Can you work these out from the model? Positions are in its coordinate system, mm. Face numbers are marked on the shaded views. Give positions to 0.01 mm unless a question says otherwise; leave off trailing zeros. Order: outer loops, then holes, each group sorted by start corner. A loop starts at its lowest first (then second) coordinate and runs counter-clockwise, first axis right, second up. Notation, with made-up numbers: M 56.5,13.5 L 110.5,13.5 A25 ccw 110.5,30.5 Z; hole C 19,19 d8. An arc over 180 degrees is marked long. Answer as a JSON object with one key per item and string values.
```python
from build123d import *

# Parameters (mm, degrees)
PAD_DEPTH    = 10
CHAMFER_SIZE = 1


with BuildPart() as part:
    # Sketch → Pad (new body)
    with BuildSketch(Plane.XY):
        with BuildLine():
            Line((-0.8, 8), (-0.8, 0))
            Line((-0.8, 0), (0.8, 0))
            Line((0.8, 8), (0.8, 0))
            ThreePointArc((3.222844, 7.624292), (2.025901, 7.905515), (0.8, 8))
            Line((3.222844, 7.624292), (68.028555, -12.969635))
            ThreePointArc((75, -22.5), (73.071107, -16.595999), (68.028555, -12.969635))
            Line((75, -22.5), (65, -22.5))
            ThreePointArc((65, -22.5), (0, -10), (-65, -22.5))
            Line((-75, -22.5), (-65, -22.5))
            ThreePointArc((-68.028555, -12.969635), (-73.071107, -16.595999), (-75, -22.5))
            Line((-3.222844, 7.624292), (-68.028555, -12.969635))
            ThreePointArc((-0.8, 8), (-2.025901, 7.905515), (-3.222844, 7.624292))
        make_face()
    extrude(amount=PAD_DEPTH)

    # Chamfer
    chamfer_edges = [part.edges().sort_by_distance(p)[0] for p in [
        (-2.025901, 7.905515, 10),
        (-0.8, 4, 10),
        (0, 0, 10),
        (0.8, 4, 10),
        (2.025901, 7.905515, 10),
        (35.625699, -2.672672, 10),
        (73.071107, -16.595999, 10),
        (70, -22.5, 10),
        (0, -10, 10),
        (-70, -22.5, 10),
        (-73.071107, -16.595999, 10),
        (-35.625699, -2.672672, 10),
        (-2.025901, 7.905515, 0),
        (-0.8, 4, 0),
        (0, 0, 0),
        (0.8, 4, 0),
        (2.025901, 7.905515, 0),
        (35.625699, -2.672672, 0),
        (73.071107, -16.595999, 0),
        (70, -22.5, 0),
        (0, -10, 0),
        (-70, -22.5, 0),
        (-73.071107, -16.595999, 0),
        (-35.625699, -2.672672, 0),
        (-0.8, 8, 5),
        (0.8, 8, 5),
        (-75, -22.5, 5),
        (-65, -22.5, 5),
        (65, -22.5, 5),
        (75, -22.5, 5),
    ]]
    chamfer(chamfer_edges, length=CHAMFER_SIZE)


solid = part.part
```
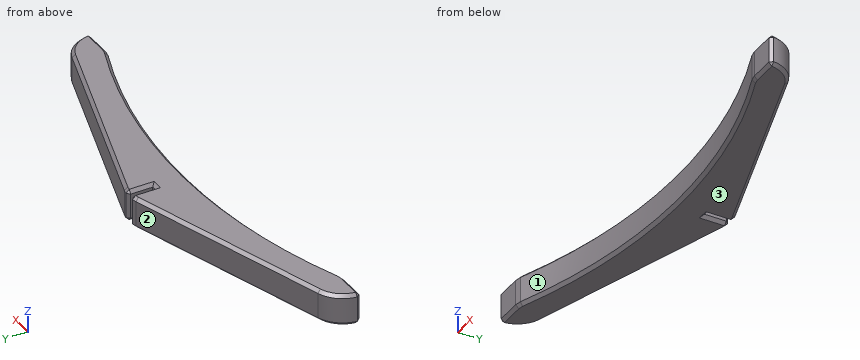
1) I need wall thicknesses on L1, parallel to Y at x = -47, z = 8.25; L2, parallel to Z at x = -35, y = -13; L3, parallel to Y at x = 48.5, z = 2.5. Which ranges of each line are inside material? Lowest first, please.
Results found:
{"L1": "y = -16.42 to -6.29", "L2": "z = 0.48 to 9.52", "L3": "y = -16.84 to -6.76"}
2) I want a section at A-A on y = 3. Write out the boundary of the cut face in (x, z).
Results found:
{"outline": "M -17.77,1 L -14.47,0 L -1.8,0 L -0.8,1 L -0.8,9 L -1.8,10 L -14.47,10 L -17.77,9 Z; M 0.8,1 L 1.8,0 L 14.47,0 L 17.77,1 L 17.77,9 L 14.47,10 L 1.8,10 L 0.8,9 Z"}
3) I want a section at B-B on z = 4. Write out the boundary of the cut face in (x, y).
Results found:
{"outline": "M -74.95,-21.5 L -74,-22.5 L -66,-22.5 L -64.07,-22.13 A175.25 cw 64.07,-22.13 L 66,-22.5 L 74,-22.5 L 74.95,-21.5 A10 ccw 68.03,-12.97 L 3.22,7.62 A8 ccw 1.8,7.94 L 0.8,7 L 0.8,0 L -0.8,0 L -0.8,7 L -1.8,7.94 A8 ccw -3.22,7.62 L -68.03,-12.97 A10 ccw Z"}
4) Thinking about a two-plate mould opening in X: for the marked faces 1, 2 and 3, which applies, pulls with the +X half, pulls with the -X half, needs draft (parallel to the pull), parting line crosses it, or undercut?
Results found:
{"face 1": "undercut", "face 2": "pulls with the -X half", "face 3": "needs draft"}
5) I'm going to push flat-ended pins straight in: pin 1 Ø3 at (y, z) = (-14.5, 6.5) entering from -X; pin 2 Ø3 at (x, z) = (53, 6) entering from +Y; pin 3 Ø1.3 at (x, z) = (0, 5) entering from +Y. Where does each tip first touch, or does it pass through?
Results found:
{"pin 1": "stops at x = -72.6", "pin 2": "stops at y = -7.72", "pin 3": "stops at y = 0"}
6) I want a section at C-C on y = -6. Write out the boundary of the cut face in (x, z).
Results found:
{"outline": "M -46.1,1 L -42.79,0 L 42.79,0 L 46.1,1 L 46.1,9 L 42.79,10 L -42.79,10 L -46.1,9 Z"}
